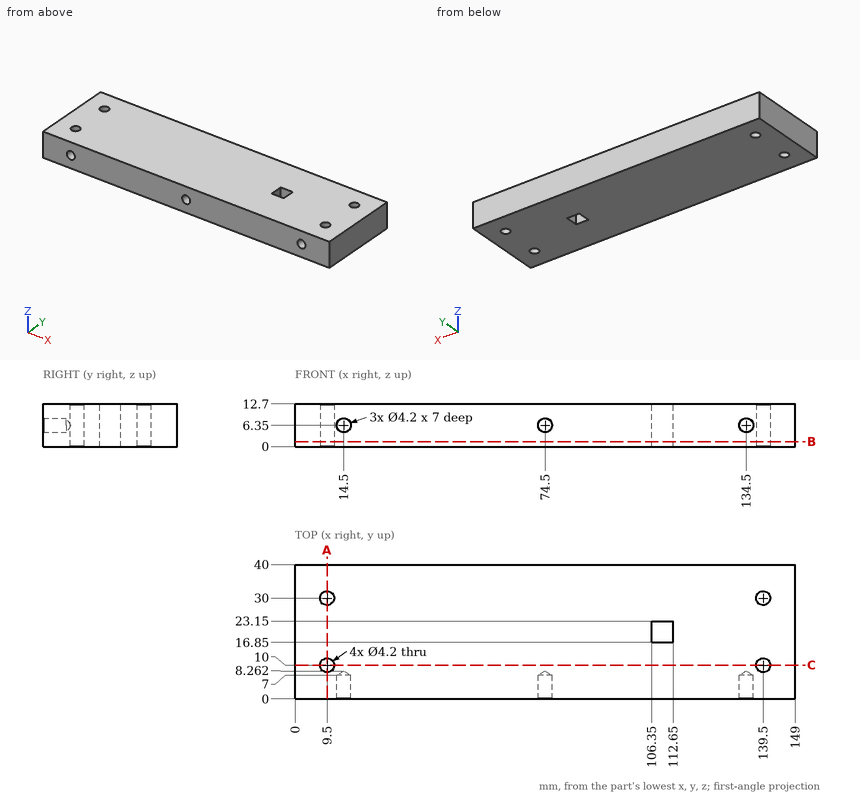
Check sheet for the drawn part. Datum: minimum x, y, z corner. Units: mm. Give positions to 0.01 mm unless a question says otherwise; leave off trailing zeros. Order: outer loops, then holes, each group sorted by start corner. A loop starts at its lowest first (then second) coordinate and runs counter-clockwise, first axis right, second up. Notation, with made-up numbers: (37, -27.5) -> (65, -27.5) arc R23 ccw to (65, -13.5) -> close; hole circle Ø2 at (-24.5, 33.5). An arc over 180 degrees is marked (long way). Return JSON: item names as keys, results as strings.
1. Cross-section at A-A, the plane x = 9.5. Record the cut outline in (y, z), plus the area to 3 significant figures.
From the geometry:
{"outline": "(0, 0) -> (7.9, 0) -> (7.9, 12.7) -> (0, 12.7) -> close; (12.1, 0) -> (27.9, 0) -> (27.9, 12.7) -> (12.1, 12.7) -> close; (32.1, 0) -> (40, 0) -> (40, 12.7) -> (32.1, 12.7) -> close", "area": "401 mm^2"}
2. Go/stop test with flat-tipped pins: P1, Ø6.5, axis at x = 139.5, y = 30, coming from the -Z side; P2, Ø3.5, axis at x = 9.5, y = 30, coming from the +Z side; P3, Ø4, axis at x = 134.5, z = 6.35, coming from the -Y side. Record where each tip stops, or that it passes through.
From the geometry:
{"P1": "z = 0", "P2": "through", "P3": "y = 7.06"}
3. Material ranges on probe 1 along Z at (x, y) = (134.5, 4.25); probe 2 along X at (y, z) = (19.5, 10.5); probe 3 along X at (y, z) = (30.5, 4.75), recorded low to high. Write a range as [from, to].
From the geometry:
{"probe 1": "[0, 4.25], [8.45, 12.7]", "probe 2": "[0, 106.35], [112.65, 149]", "probe 3": "[0, 7.46], [11.54, 137.46], [141.54, 149]"}
4. Cross-section at C-C, the plane y = 10. Record the cut outline in (x, z).
From the geometry:
{"outline": "(0, 0) -> (7.4, 0) -> (7.4, 12.7) -> (0, 12.7) -> close; (11.6, 0) -> (137.4, 0) -> (137.4, 12.7) -> (11.6, 12.7) -> close; (141.6, 0) -> (149, 0) -> (149, 12.7) -> (141.6, 12.7) -> close"}
5. Cross-section at B-B, the plane z = 1.5. Record the cut outline in (x, y), plus the area to 4 significant figures.
From the geometry:
{"outline": "(0, 0) -> (149, 0) -> (149, 40) -> (0, 40) -> close; hole circle Ø4.2 at (9.5, 10); hole circle Ø4.2 at (9.5, 30); hole (106.35, 16.85) -> (112.65, 16.85) -> (112.65, 23.15) -> (106.35, 23.15) -> close; hole circle Ø4.2 at (139.5, 10); hole circle Ø4.2 at (139.5, 30)", "area": "5,865 mm^2"}
